Answer from the drawing. Dimensions are ordinates in mm from the lowest x, y and z of the part. Coordinates: 2 decimals unless noted, no trailing zeros. Write each loop counter-clockwise with the first axis right and the second up, starting at its lowest first coordinate (ties: lowest second). Pieces come first, ordered by that corner, then holes. Notation, with made-up numbers: (55.25, 54.5) - (65.25, 54.5) arc R10 ccw to (65.25, 73.5) - close; hole circle Ø6 at (49.5, 2.25). An arc over 180 degrees is marked (long way). Use a Markdown table: item, result.
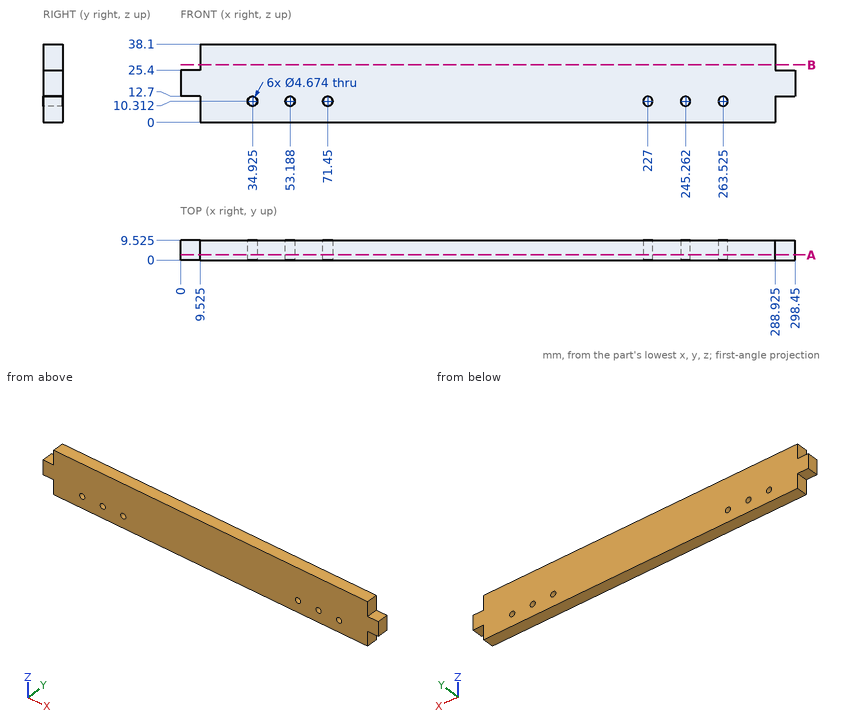
(1) Each of these flat-tipped pins is pushed along its axis until it touches: P1, Ø3.5, axis at x = 263.52, z = 10.31, coming from the -Y side; P2, Ø5, axis at x = 5.5, y = 6.5, coming from the +Z side; P3, Ø3, axis at y = 6, z = 7.5, coming from the +X side (3 decimals). Where does it stop, or does it pass through?
Report:
| item | result |
|---|---|
| P1 | passes through |
| P2 | stops at z = 25.4 |
| P3 | stops at x = 288.925 |
(2) Straight lines are drawn through the part: L1, parallel to Z at x = 70, y = 2 (1 decimal); L2, parallel to X at y = 2.75, z = 4.5 (1 decimal). For each, find the intervals that lie inside material, in ascending order.
Report:
| item | result |
|---|---|
| L1 | z = 0 to 8.5, 12.1 to 38.1 |
| L2 | x = 9.5 to 288.9 |
(3) A cutting plane is placed at A-A, the plane y = 2.5. Count the separate pieces of the cut face and the enclosed holes in it, and give its area (3 significant figures).
Report:
| item | result |
|---|---|
| separate pieces | 1 |
| enclosed holes | 6 |
| area | 10,800 mm² |
(4) A cutting plane is placed at B-B, the plane z = 28. Write down the section's boundary in (x, y) (1 decimal), and give its area (3 significant figures).
Report:
| item | result |
|---|---|
| outline | (9.5, 0) - (288.9, 0) - (288.9, 9.5) - (9.5, 9.5) - close |
| area | 2,660 mm² |
